from build123d import *
from build123d.topology import SkipClean

# Parameters (mm, degrees)
SKETCH1_R           = 49.53
SKETCH1_R_2         = 34.29
BOSS_EXTRUDE1_DEPTH = 6.35
SKETCH2_R           = 2.5527
BOSS_EXTRUDE2_DEPTH = 177.8
SKETCH5_R           = 2.5527
CUT_EXTRUDE1_DEPTH  = 6.35
BOSS_EXTRUDE3_START = -6.35
SKETCH2_3_R         = 2.5527
BOSS_EXTRUDE3_DEPTH = 6.35


with BuildPart() as part:
    # Sketch1 → Boss-Extrude1 (new body)
    with BuildSketch(Plane(origin=(0, 0, 0), x_dir=(1, 0, 0), z_dir=(0, 1, 0))):
        with Locations(Location((0, 0, 0), (0, 0, 270))):
            Circle(SKETCH1_R)
        with Locations(Location((0, 0, 0), (0, 0, 270))):
            Circle(SKETCH1_R_2, mode=Mode.SUBTRACT)
    extrude(amount=BOSS_EXTRUDE1_DEPTH)

    # Sketch2 → Boss-Extrude2 (add)
    # profile 1 of 2: a face of its own
    with SkipClean():  # the faces are left unmerged after this step: merging them gives an invalid solid
        with BuildSketch(Plane(origin=(0, 6.35, 0), x_dir=(1, 0, 0), z_dir=(0, 1, 0))):
            with BuildLine():
                Line((-49.106263984, 6.464962301), (-33.996644297, 4.475743131))
                ThreePointArc((-33.996644297, 4.475743131), (-30.819076289, 0), (-33.996644297, -4.475743131))
                Line((-33.996644297, -4.475743131), (-49.106263984, -6.464962301))
                ThreePointArc((-49.106263984, -6.464962301), (-49.53, 0), (-49.106263984, 6.464962301))
            make_face()
            with Locations(Location((-35.56, 0, 0), (0, 0, 58.363987486))):
                Circle(SKETCH2_R, mode=Mode.SUBTRACT)
        # profile 2 of 2: a face of its own
        with BuildSketch(Plane(origin=(0, 6.35, 0), x_dir=(1, 0, 0), z_dir=(0, 1, 0))):
            with BuildLine():
                Line((33.996644297, 4.475743131), (49.106263984, 6.464962301))
                ThreePointArc((49.106263984, 6.464962301), (49.53, 0), (49.106263984, -6.464962301))
                Line((49.106263984, -6.464962301), (33.996644297, -4.475743131))
                ThreePointArc((33.996644297, -4.475743131), (30.819076289, 0), (33.996644297, 4.475743131))
            make_face()
            with Locations(Location((35.56, 0, 0), (0, 0, 90))):
                Circle(SKETCH2_R, mode=Mode.SUBTRACT)
        extrude(amount=BOSS_EXTRUDE2_DEPTH)

    # Sketch5 → Cut-Extrude1 (cut)
    with SkipClean():  # the faces are left unmerged after this step: merging them gives an invalid solid
        with BuildSketch(Plane.XZ):
            with Locations(Location((-35.56, 0, 0), (0, 0, 301.636012514))):
                Circle(SKETCH5_R)
            with Locations(Location((35.56, 0, 0), (0, 0, 270))):
                Circle(SKETCH5_R)
        extrude(amount=-CUT_EXTRUDE1_DEPTH, mode=Mode.SUBTRACT)

    # Sketch2_3 → Boss-Extrude3 (add)
    # profile 1 of 2: a face of its own
    with BuildSketch(Plane(origin=(0, 6.35, 0), x_dir=(1, 0, 0), z_dir=(0, 1, 0)).offset(BOSS_EXTRUDE3_START)):
        with BuildLine():
            Line((-49.106263984, 6.464962301), (-33.996644297, 4.475743131))
            ThreePointArc((-33.996644297, 4.475743131), (-30.819076289, 0), (-33.996644297, -4.475743131))
            Line((-33.996644297, -4.475743131), (-49.106263984, -6.464962301))
            ThreePointArc((-49.106263984, -6.464962301), (-49.53, 0), (-49.106263984, 6.464962301))
        make_face()
        with Locations(Location((-35.56, 0, 0), (0, 0, 90))):
            Circle(SKETCH2_3_R, mode=Mode.SUBTRACT)
    # profile 2 of 2: a face of its own
    with BuildSketch(Plane(origin=(0, 6.35, 0), x_dir=(1, 0, 0), z_dir=(0, 1, 0)).offset(BOSS_EXTRUDE3_START)):
        with BuildLine():
            Line((33.996644297, 4.475743131), (49.106263984, 6.464962301))
            ThreePointArc((49.106263984, 6.464962301), (49.53, 0), (49.106263984, -6.464962301))
            Line((49.106263984, -6.464962301), (33.996644297, -4.475743131))
            ThreePointArc((33.996644297, -4.475743131), (30.819076289, 0), (33.996644297, 4.475743131))
        make_face()
        with Locations(Location((35.56, 0, 0), (0, 0, 90))):
            Circle(SKETCH2_3_R, mode=Mode.SUBTRACT)
    extrude(amount=BOSS_EXTRUDE3_DEPTH)


solid = part.part
Read the model definition and answer for the solid it produces. Units are mm, in the model's axes. A direction names the side the tool comes from. Coordinates: 2 decimals unless noted, no trailing zeros. Loops run counter-clockwise (first coordinate to the right, second up) from the corner with the lowest first, then second, coordinate; pieces in that order, holes last. Notation, with made-up numbers: (28, 45.25) -> (51, 45.25) arc R21 cw to (51, 63.25) -> close; hole circle Ø8 at (31, 60.5). An arc over 180 degrees is marked (long way). Answer in a Markdown table with one row per item.
Item 1: A cutting plane is placed at D-D on z = -21. Determine the outline of the cut face in (x, y).
Returned:
| item | result |
|---|---|
| outline | (-44.86, 0) -> (-27.11, 0) -> (-27.11, 6.35) -> (-44.86, 6.35) -> close; (27.11, 0) -> (44.86, 0) -> (44.86, 6.35) -> (27.11, 6.35) -> close |
Item 2: Each of these flat-tipped pins is pushed along its axis until it touches: P1, Ø1, axis at x = 28.5, z = 20.5, coming from the -Y side; P2, Ø4.5, axis at x = -35.56, z = 0, coming from the +Y side. Where does it stop, or does it pass through?
Returned:
| item | result |
|---|---|
| P1 | stops at y = 0 |
| P2 | passes through |
Item 3: For faces 3 (the flat face through (41.446, 94.005, -5.456)), 4 (the flat face through (-41.446, 94.005, 5.456)), 5 (the cylindrical face through (0.691, 3.131, -34.283)), 6 (the flat face through (-32, 0, -1)), determine the directions among +Z, -Z, +X, -X, +Y, -Y from which every point of the face is accessible in a straight line to the end or side of a thin tool.
Returned:
| item | result |
|---|---|
| face 3 | -Z, +Y |
| face 4 | +Z, +Y |
| face 5 | +Y, -Y |
| face 6 | +Z, -Z, +X, -X, -Y |
Item 4: For a pull along X with two mould halves and no side action, classify faces 1 (the flat face through (-41.657, 94.005, -5.484)), 2 (the flat face through (42, 184.15, 0)) as released by +X, released by -X, zero draft, split by the parting line, or undercut.
Returned:
| item | result |
|---|---|
| face 1 | undercut |
| face 2 | zero draft |
Item 5: A cutting plane is placed at A-A on z = 0. Determine the outline of the cut face in (x, y), plus the area to 3 significant figures.
Returned:
| item | result |
|---|---|
| outline | (-49.53, 0) -> (-38.11, 0) -> (-38.11, 184.15) -> (-49.53, 184.15) -> close; (-33.01, 0) -> (-30.82, 0) -> (-30.82, 184.15) -> (-33.01, 184.15) -> close; (30.82, 0) -> (33.01, 0) -> (33.01, 184.15) -> (30.82, 184.15) -> close; (38.11, 0) -> (49.53, 0) -> (49.53, 184.15) -> (38.11, 184.15) -> close |
| area | 5,010 mm^2 |
Item 6: Straight lines are drawn through the part: line 1 along X through (y, z) = (53, 0); line 2 along X through (y, z) = (42, -2); line 3 along Y through (x, z) = (9, 40). For each, find the intervals that lie inside material, in ascending order. Write a range as [from, to].
Returned:
| item | result |
|---|---|
| line 1 | x = [-49.53, -38.11], [-33.01, -30.82], [30.82, 33.01], [38.11, 49.53] |
| line 2 | x = [-49.49, -37.15], [-33.97, -31.26], [31.26, 33.97], [37.15, 49.49] |
| line 3 | y = [0, 6.35] |
Item 7: A cutting plane is placed at C-C on x = -12.5. Determine the outline of the cut face in (y, z), plus the area to 3 significant figures.
Returned:
| item | result |
|---|---|
| outline | (0, -47.93) -> (6.35, -47.93) -> (6.35, -31.93) -> (0, -31.93) -> close; (0, 31.93) -> (6.35, 31.93) -> (6.35, 47.93) -> (0, 47.93) -> close |
| area | 203 mm^2 |
Item 8: A cutting plane is placed at B-B on y = 54. Determine the outline of the cut face in (x, z).
Returned:
| item | result |
|---|---|
| outline | (-49.11, -6.46) -> (-34, -4.48) arc R4.74 ccw to (-34, 4.48) -> (-49.11, 6.46) arc R49.53 ccw to start; (34, -4.48) -> (49.11, -6.46) arc R49.53 ccw to (49.11, 6.46) -> (34, 4.48) arc R4.74 ccw to start; hole circle Ø5.11 at (-35.56, 0); hole circle Ø5.11 at (35.56, 0) |
